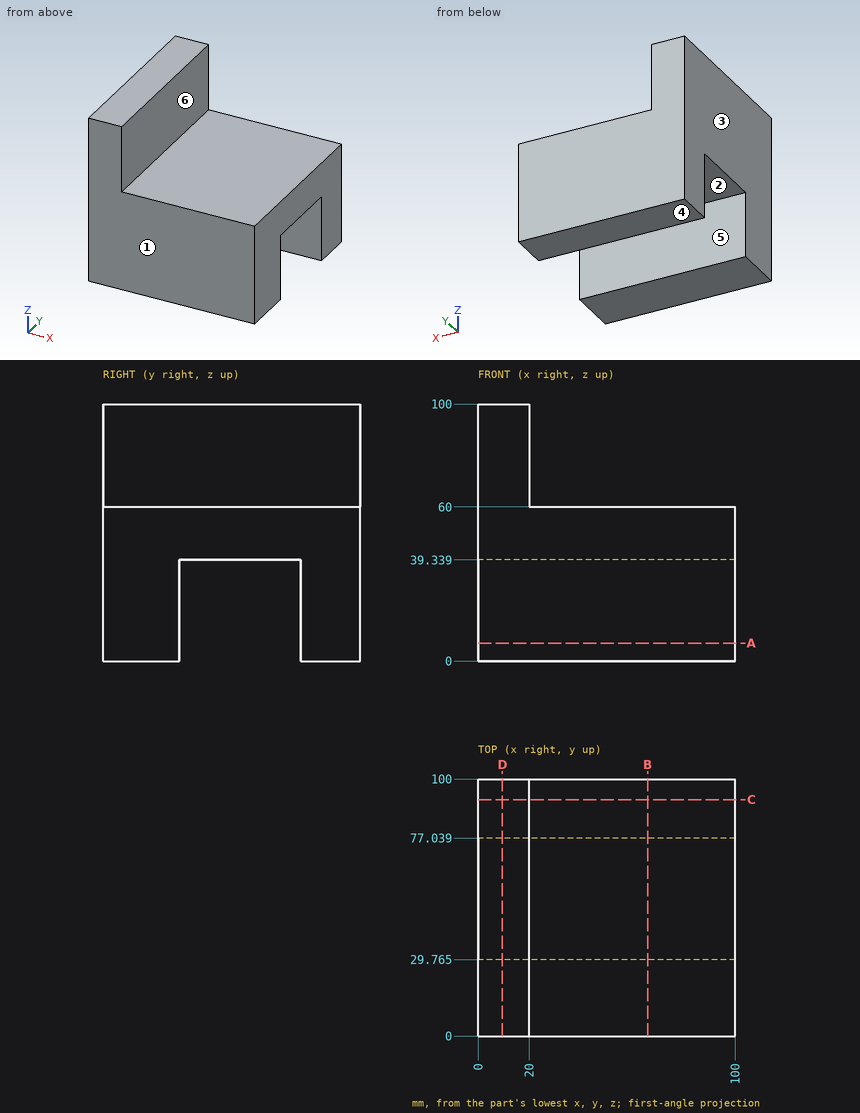
For this review, use the dimensioned drawing (mm, ordinates from the lowest corner) and the shaded views. A direction names the side the tool comes from. Coordinates: 2 decimals unless noted, no trailing zeros. Order: outer loops, then holes, each group sorted by start corner. A loop starts at its lowest first (then second) coordinate and runs counter-clockwise, first axis right, second up. Notation, with made-up numbers: (35, -23) - (70, -23) arc R16 ccw to (70, -3) - close; hole circle Ø6 at (7.5, 81). An arc over 180 degrees is marked (long way). Use one line per item in the form item = value.
Q1. For the marked faces 4, 5 and 6, list the 3-axis set-ups (+Z, -Z, +X, -X, +Y, -Y) from which the entire face can be reached by the end or side of a thin tool; tool diameter is ignored.
Checked values:
face_4 = -Z, +X, -X, +Y, -Y
face_5 = -Z, +X, -X
face_6 = +Z, +X, +Y, -Y
Q2. Consider section A-A (z = 7). Give the boundary of the cut face in (x, y) (1 decimal).
Checked values:
outline = (0, 0) - (100, 0) - (100, 29.8) - (0, 29.8) - close; (0, 77) - (100, 77) - (100, 100) - (0, 100) - close
Q3. For probe 1 along Y at (x, z) = (53.5, 32) (1 decimal); probe 2 along Z at (x, y) = (95.5, 16); probe 3 along Z at (x, y) = (50.5, 64.5), list the stretches that pass through material, from the lowest coordinate up. Write a range as from..to.
Checked values:
probe_1 = 0..29.8, 77..100
probe_2 = 0..60
probe_3 = 39.34..60
Q4. Consider section B-B (x = 66). Give the boundary of the cut face in (y, z) (1 decimal).
Checked values:
outline = (0, 0) - (29.8, 0) - (29.8, 39.3) - (77, 39.3) - (77, 0) - (100, 0) - (100, 60) - (0, 60) - close
Q5. For P1, Ø3, axis at x = 27.5, y = 46, coming from the +Z side; P2, Ø23.5, axis at x = 67.5, y = 60.5, coming from the -Z side, all flat-tipped, find the tip position at first contact; note any pin that passes through.
Checked values:
P1 = 60
P2 = 39.34
Q6. Consider section D-D (x = 9.5). Give the boundary of the cut face in (y, z) (1 decimal).
Checked values:
outline = (0, 0) - (29.8, 0) - (29.8, 39.3) - (77, 39.3) - (77, 0) - (100, 0) - (100, 100) - (0, 100) - close
Q7. Consider section C-C (y = 92). Give the boundary of the cut face in (x, z), then the cut area to 3 significant figures.
Checked values:
outline = (0, 0) - (100, 0) - (100, 60) - (20, 60) - (20, 100) - (0, 100) - close
area = 6,800 mm2
Q8. Draft analysis for pull direction Y (two halves, no side actions). For the marked faces 1, 2 and 3, state which applies: +Y half, -Y half, draft (parallel to the pull), parting line (faces both ways), or undercut.
Checked values:
face_1 = -Y half
face_2 = undercut
face_3 = draft
